Study the drawing (mm; zero at the part's minimum x, y, z) and answer. A direction names the side the tool comes from. Give positions to 0.01 mm unless a question says otherwise; leave off trailing zeros. Write each loop counter-clockwise with the first axis right and the second up, starting at its lowest first coordinate (ties: lowest second). Pieces come first, ordered by that corner, then holes. Notation, with made-up numbers: (12, 35.5) -> (24, 35.5) arc R31 ccw to (24, 69.5) -> close; hole circle Ø7 at (-23, 25.25). An arc over 180 degrees is marked (long way). One line per question, with ' | ' between items.
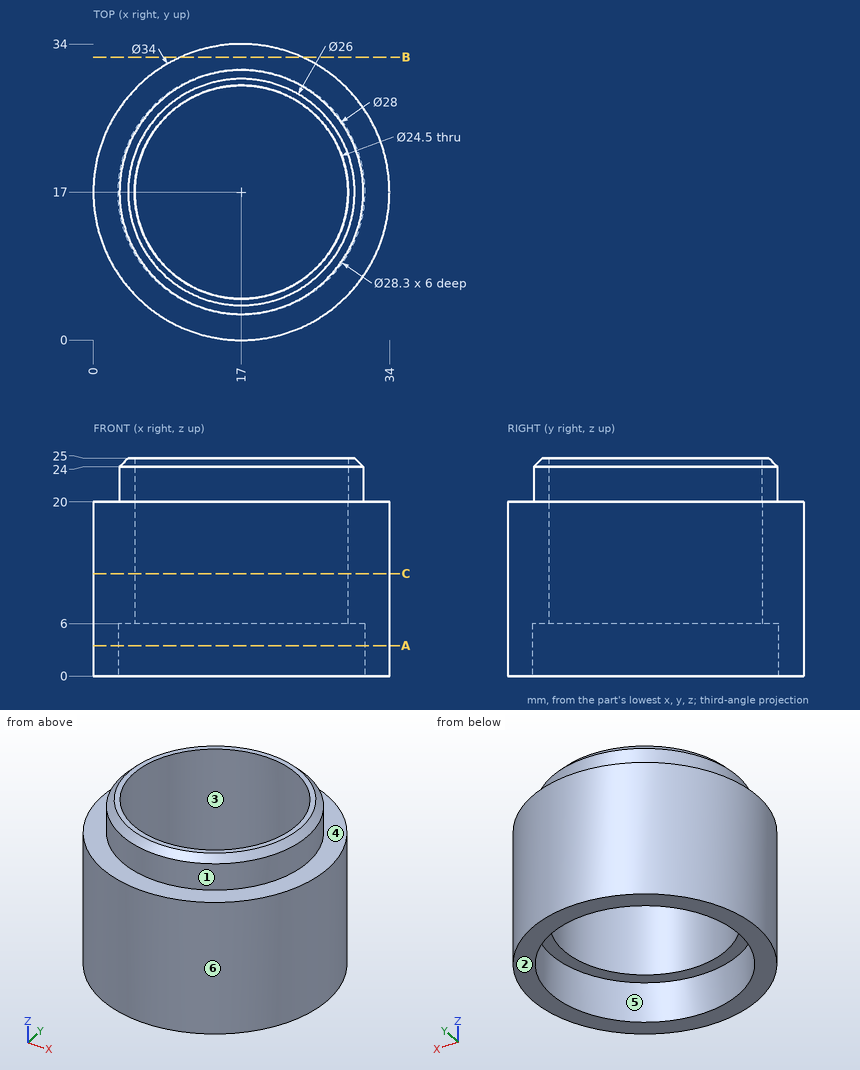
Item 1: Determine the mould class of the marked faces 3, 4, 5 and 6 for opening direction Y: pulls with the +Y half, pulls with the -Y half, needs draft (parallel to the pull), parting line crosses it, or undercut.
Answers below:
face 3: undercut | face 4: needs draft | face 5: undercut | face 6: parting line crosses it
Item 2: Flat-ended cylindrical pins translate along their axes: pin 1 (1 mm diameter, centred on y = 18, z = 17, fed in from -X); pin 2 (1.5 mm diameter, centred on x = 26, z = 9.5, fed in from -Y); pin 3 (4 mm diameter, centred on x = 29.5, z = 4, fed in from -Y). Find the tip coordinate at first contact, or state that the pin passes through.
Answers below:
pin 1: x = 0.01 | pin 2: y = 2.14 | pin 3: y = 3.63
Item 3: Find section A-A (z = 3.5). Write down the section's boundary in (x, y), then the cut area to 3 significant figures.
Answers below:
outline: circle Ø34 at (17, 17); hole circle Ø28.3 at (17, 17) | area: 279 mm²
Item 4: Find section B-B (y = 32.5). Write down the section's boundary in (x, z).
Answers below:
outline: (10.02, 0) -> (23.98, 0) -> (23.98, 20) -> (10.02, 20) -> close
Item 5: Find section C-C (z = 11.75). Write down the section's boundary in (x, y).
Answers below:
outline: circle Ø34 at (17, 17); hole circle Ø24.5 at (17, 17)
Item 6: Consider line 1 (Y direction, x = 17, z = 17.5); line 2 (Z direction, x = 4.5, y = 10); line 3 (Y direction, x = 12.5, z = 12). Determine where each line is inside the solid, lowest interval first. Write a range as [from, to].
Answers below:
line 1: [0, 4.75], [29.25, 34] | line 2: [0, 20] | line 3: [0.61, 5.61], [28.39, 33.39]
Item 7: A tool of negligible diameter and unlimited length cuts with its end or side. For the marked faces 1 and 2, from which of +Z, -Z, +X, -X, +Y, -Y can it reach the whole face along a straight path? Write none if from no direction.
Answers below:
face 1: +Z | face 2: -Z, +X, -X, +Y, -Y
